from build123d import *

# Parameters (mm, degrees)
CROQUIS1_R              = 8.5
SALIENTE_EXTRUIR1_DEPTH = 2
CROQUIS2_R              = 7.5
SALIENTE_EXTRUIR2_DEPTH = 4
CROQUIS3_R              = 15
SALIENTE_EXTRUIR3_DEPTH = 2.5
REDONDEO1_R             = 3
CORTAR_EXTRUIR1_DEPTH   = 2.5
CROQUIS5_R              = 8.5
CORTAR_EXTRUIR2_DEPTH   = 10


with BuildPart() as part:
    # Croquis1 → Saliente-Extruir1 (new body)
    with BuildSketch(Plane(origin=(0, 0, 0), x_dir=(1, 0, 0), z_dir=(0, 1, 0))):
        with Locations(Location((0, 0, 0), (0, 0, 270))):
            Circle(CROQUIS1_R)
    extrude(amount=SALIENTE_EXTRUIR1_DEPTH)

    # Croquis2 → Saliente-Extruir2 (add)
    with BuildSketch(Plane(origin=(0, 2, 0), x_dir=(1, 0, 0), z_dir=(0, 1, 0))):
        with Locations(Location((0, 0, 0), (0, 0, 270))):
            Circle(CROQUIS2_R)
    extrude(amount=SALIENTE_EXTRUIR2_DEPTH)

    # Croquis3 → Saliente-Extruir3 (add)
    with BuildSketch(Plane(origin=(0, 6, 0), x_dir=(1, 0, 0), z_dir=(0, 1, 0))):
        with Locations(Location((0, 0, 0), (0, 0, 270))):
            Circle(CROQUIS3_R)
    extrude(amount=SALIENTE_EXTRUIR3_DEPTH)

    # Redondeo1
    # the kernel refuses this fillet: 3 mm, written as the material it takes off along each edge
    with BuildSketch(Plane(origin=(0, 0, 0), x_dir=(0, 0, 1), z_dir=(-1, 0, 0))) as redondeo1_piece_1:
        with BuildLine():
            CenterArc((5.671572875, 3), REDONDEO1_R, 270, 70.528779366)
            Line((5.671572875, 0), (5.671572875, -0.06))
            Line((5.671572875, -0.06), (8.5, -0.06))
            Line((8.5, -0.06), (8.56, 0))
            ThreePointArc((8.56, 0), (8.56, 1), (8.556568542, 1.98))
            Line((8.556568542, 1.98), (8.5, 2))
        make_face()
    revolve(axis=Axis((0, 0, 0), (0, 1, 0)), mode=Mode.SUBTRACT)

    # Croquis4 → Cortar-Extruir1 (cut)
    with BuildSketch(Plane(origin=(0, 8.5, 0), x_dir=(1, 0, 0), z_dir=(0, 1, 0))):
        Polygon((12.154001459, -1.732050808), (12.154001459, 1.732050808), (9.154001459, 3.464101615), (6.154001459, 1.732050808), (6.154001459, -1.732050808), (9.154001459, -3.464101615), align=None)
        Polygon((3.464101615, 9.154001459), (1.732050808, 12.154001459), (-1.732050808, 12.154001459), (-3.464101615, 9.154001459), (-1.732050808, 6.154001459), (1.732050808, 6.154001459), align=None)
        Polygon((-1.732050808, -12.154001459), (1.732050808, -12.154001459), (3.464101615, -9.154001459), (1.732050808, -6.154001459), (-1.732050808, -6.154001459), (-3.464101615, -9.154001459), align=None)
        Polygon((-12.154001459, 1.732050808), (-12.154001459, -1.732050808), (-9.154001459, -3.464101615), (-6.154001459, -1.732050808), (-6.154001459, 1.732050808), (-9.154001459, 3.464101615), align=None)
    extrude(amount=-CORTAR_EXTRUIR1_DEPTH, mode=Mode.SUBTRACT)

    # Croquis5 → Cortar-Extruir2 (cut)
    with BuildSketch(Plane.XZ.offset(-6)):
        Circle(CROQUIS5_R)
    extrude(amount=CORTAR_EXTRUIR2_DEPTH, mode=Mode.SUBTRACT)


solid = part.part
Work out the finished part from the listing and answer in its coordinate system (mm). A direction names the side the tool comes from. Coordinates: 2 decimals unless noted, no trailing zeros. Loops run counter-clockwise (first coordinate to the right, second up) from the corner with the lowest first, then second, coordinate; pieces in that order, holes last. Notation, with made-up numbers: (40, 43.25) -> (86, 43.25) arc R14 cw to (86, 60.25) -> close; hole circle Ø8 at (-30.75, 81.5). An arc over 180 degrees is marked (long way). Answer as CSV lines item,"result".
1) The part is cut by section B-B (z = 0). Give the vertices of the cut face in (x, y).
A:
outline,"(-15, 6) -> (-12.15, 6) -> (-12.15, 8.5) -> (-15, 8.5) -> close; (-6.15, 6) -> (6.15, 6) -> (6.15, 8.5) -> (-6.15, 8.5) -> close; (12.15, 6) -> (15, 6) -> (15, 8.5) -> (12.15, 8.5) -> close"
2) For faces 4 (the face through (6.154, 7, 0)), 5 (the face through (0, 6, 0)), determine the directions among +Z, -Z, +X, -X, +Y, -Y from which every point of the face is accessible in a straight line to the end or side of a thin tool.
A:
face 4,"+Y, -Y"
face 5,"+Z, -Z, +X, -X, -Y"
3) For a pull along X with two mould halves and no side action, classify faces 1 (the face through (12.154, 7, 0)), 2 (the face through (0, 8.5, 0)), 3 (the face through (0.66, 7.232, -14.985)) as released by +X, released by -X, zero draft, split by the parting line, or undercut.
A:
face 1,"undercut"
face 2,"zero draft"
face 3,"split by the parting line"
4) Straight lines are drawn through the part: probe 1 along Z at (x, y) = (-0.5, 7.75); probe 2 along X at (y, z) = (7.3, 2.5); probe 3 along X at (y, z) = (6.6, 1). For each, find the intervals that lie inside material, in ascending order.
A:
probe 1,"z = -14.99 to -12.15, -6.15 to 6.15, 12.15 to 14.99"
probe 2,"x = -14.79 to -10.82, -7.48 to 7.48, 10.82 to 14.79"
probe 3,"x = -14.97 to -12.15, -6.15 to 6.15, 12.15 to 14.97"
5) Flat-ended cylindrical pins translate along their axes: pin 1 (1 mm diameter, centred on y = 8, z = 6, fed in from +X); pin 2 (0.8 mm diameter, centred on y = 8, z = 1, fed in from -X); pin 3 (1.2 mm diameter, centred on y = 7, z = -0.5, fed in from +X); pin 4 (1 mm diameter, centred on x = -5.5, y = 7.5, fed in from -Z). Find the tip coordinate at first contact, or state that the pin passes through.
A:
pin 1,"stops at x = 13.96"
pin 2,"stops at x = -14.99"
pin 3,"stops at x = 15"
pin 4,"stops at z = -14.14"
6) The part is cut by section A-A (x = 0). Give the vertices of the cut face in (y, z), and give its area (3 significant figures).
A:
outline,"(6, -15) -> (8.5, -15) -> (8.5, -12.15) -> (6, -12.15) -> close; (6, -6.15) -> (8.5, -6.15) -> (8.5, 6.15) -> (6, 6.15) -> close; (6, 12.15) -> (8.5, 12.15) -> (8.5, 15) -> (6, 15) -> close"
area,"45.0 mm²"
7) The part is cut by section C-C (y = 7.75). Give the vertices of the cut face in (x, z).
A:
outline,"circle Ø30 at (0, 0); hole (-12.15, -1.73) -> (-9.15, -3.46) -> (-6.15, -1.73) -> (-6.15, 1.73) -> (-9.15, 3.46) -> (-12.15, 1.73) -> close; hole (-3.46, -9.15) -> (-1.73, -12.15) -> (1.73, -12.15) -> (3.46, -9.15) -> (1.73, -6.15) -> (-1.73, -6.15) -> close; hole (-3.46, 9.15) -> (-1.73, 6.15) -> (1.73, 6.15) -> (3.46, 9.15) -> (1.73, 12.15) -> (-1.73, 12.15) -> close; hole (6.15, -1.73) -> (9.15, -3.46) -> (12.15, -1.73) -> (12.15, 1.73) -> (9.15, 3.46) -> (6.15, 1.73) -> close"
8) The part is cut by section D-D (x = -6.5). Give the vertices of the cut face in (y, z), and give its area (3 significant figures).
A:
outline,"(6, -13.52) -> (8.5, -13.52) -> (8.5, -1.93) -> (6, -1.93) -> close; (6, 1.93) -> (8.5, 1.93) -> (8.5, 13.52) -> (6, 13.52) -> close"
area,"57.9 mm²"
